Verification items for the finished model (mm, model axes). A direction names the side the tool comes from. Coordinates: 2 decimals unless noted, no trailing zeros. Write each loop counter-clockwise with the first axis right and the second up, starting at its lowest first coordinate (ties: lowest second). Pieces come first, ordered by that corner, then holes. Notation, with made-up numbers: M -15.75,-40 L 26.25,-40 A12 cw 26.25,-18 Z; hole C 71.5,-1 d10. An arc over 180 degrees is marked long. One line per item, written item: value.
```python
from build123d import *

# Parameters (mm, degrees)
CROQUIS1_W                 = 45
CROQUIS1_H                 = 45
SALIENTE_EXTRUIR1_DEPTH    = 300
CROQUIS4_W                 = 18
CROQUIS4_H                 = 34
CORTAR_EXTRUIR2_DEPTH      = 46
CROQUIS8_W                 = 35
CROQUIS8_H                 = 35
CORTAR_EXTRUIR3_DEPTH      = 301
CROQUIS9_W                 = 35
CROQUIS9_H                 = 21.174410022
CORTAR_EXTRUIR4_DEPTH      = 10
CROQUIS10_R                = 1
CORTAR_EXTRUIR5_DEPTH      = 10
CROQUIS11_W                = 45
CROQUIS11_H                = 26.387879272
CORTAR_EXTRUIR6_DEPTH      = 46
CROQUIS13_W                = 45
CROQUIS13_H                = 50
CORTAR_EXTRUIR7_DEPTH      = 23.5
CORTAR_EXTRUIR7_DEPTH_BACK = 23.5
CROQUIS14_W                = 55
CROQUIS14_H                = 55
SALIENTE_EXTRUIR2_DEPTH    = 5
CROQUIS16_R                = 1
CORTAR_EXTRUIR8_DEPTH      = 1
CORTAR_EXTRUIR8_DEPTH_BACK = 229.612120728
CROQUIS17_R                = 2.5
CROQUIS17_R_2              = 2.03
CROQUIS17_R_3              = 1.793308219
CORTAR_EXTRUIR9_DEPTH      = 6
CORTAR_EXTRUIR9_DEPTH_BACK = 51


with BuildPart() as part:
    # Croquis1 → Saliente-Extruir1 (new body)
    with BuildSketch(Plane(origin=(0, 0, 0), x_dir=(1, 0, 0), z_dir=(0, 1, 0))):
        Rectangle(CROQUIS1_W, CROQUIS1_H)
    extrude(amount=SALIENTE_EXTRUIR1_DEPTH)

    # Croquis4 → Cortar-Extruir2 (cut, through all)
    with BuildSketch(Plane.ZY.offset(22.5)):
        with Locations((13.5, 17)):
            Rectangle(CROQUIS4_W, CROQUIS4_H)
    extrude(amount=-CORTAR_EXTRUIR2_DEPTH, mode=Mode.SUBTRACT)

    # Croquis8 → Cortar-Extruir3 (cut, through all)
    with BuildSketch(Plane(origin=(0, 300, 0), x_dir=(1, 0, 0), z_dir=(0, 1, 0))):
        Rectangle(CROQUIS8_W, CROQUIS8_H)
    extrude(amount=-CORTAR_EXTRUIR3_DEPTH, mode=Mode.SUBTRACT)

    # Croquis9 → Cortar-Extruir4 (cut)
    with BuildSketch(Plane(origin=(0, 0, -22.5), x_dir=(-1, 0, 0), z_dir=(0, 0, -1))):
        with Locations((0, 260)):
            Rectangle(CROQUIS9_W, CROQUIS9_H)
    extrude(amount=-CORTAR_EXTRUIR4_DEPTH, mode=Mode.SUBTRACT)

    # Croquis10 → Cortar-Extruir5 (cut)
    with BuildSketch(Plane.XY.offset(22.5)):
        with Locations((0, 260)):
            Circle(CROQUIS10_R)
    extrude(amount=-CORTAR_EXTRUIR5_DEPTH, mode=Mode.SUBTRACT)

    # Croquis11 → Cortar-Extruir6 (cut, through all)
    with BuildSketch(Plane.XY.offset(22.5)):
        with Locations((0, 286.806060364)):
            Rectangle(CROQUIS11_W, CROQUIS11_H)
    extrude(amount=-CORTAR_EXTRUIR6_DEPTH, mode=Mode.SUBTRACT)

    # Croquis13 → Cortar-Extruir7 (cut, two sides)
    with BuildSketch(Plane(origin=(0, 0, 0), x_dir=(0, 0, -1), z_dir=(1, 0, 0))) as cortar_extruir7_sk:
        with Locations((0, 25)):
            Rectangle(CROQUIS13_W, CROQUIS13_H)
    extrude(amount=CORTAR_EXTRUIR7_DEPTH, mode=Mode.SUBTRACT)
    extrude(cortar_extruir7_sk.sketch, amount=-CORTAR_EXTRUIR7_DEPTH_BACK, mode=Mode.SUBTRACT)

    # Croquis14 → Saliente-Extruir2 (add)
    with BuildSketch(Plane.XZ.offset(-50)):
        Rectangle(CROQUIS14_W, CROQUIS14_H)
    extrude(amount=SALIENTE_EXTRUIR2_DEPTH)

    # Croquis16 → Cortar-Extruir8 (cut, two sides)
    with BuildSketch(Plane.XZ.offset(-45)) as cortar_extruir8_sk:
        with Locations((25, 25)):
            Circle(CROQUIS16_R)
        with Locations((-25, 25)):
            Circle(CROQUIS16_R)
        with Locations((-25, -25)):
            Circle(CROQUIS16_R)
        with Locations((25, -25)):
            Circle(CROQUIS16_R)
    extrude(amount=CORTAR_EXTRUIR8_DEPTH, mode=Mode.SUBTRACT)
    extrude(cortar_extruir8_sk.sketch, amount=-CORTAR_EXTRUIR8_DEPTH_BACK, mode=Mode.SUBTRACT)

    # Croquis17 → Cortar-Extruir9 (cut, two sides)
    with BuildSketch(Plane.XY.offset(22.5)) as cortar_extruir9_sk:
        with Locations((-10, 262.50260741)):
            Circle(CROQUIS17_R)
        with Locations((-10, 254.10260741)):
            Circle(CROQUIS17_R_2)
        with Locations((-10, 214.90260741)):
            Circle(CROQUIS17_R_3)
        with Locations((-10, 206.50260741)):
            Circle(CROQUIS17_R)
        with Locations((10, 262.50260741)):
            Circle(CROQUIS17_R)
        with Locations((10, 206.50260741)):
            Circle(CROQUIS17_R)
    extrude(amount=CORTAR_EXTRUIR9_DEPTH, mode=Mode.SUBTRACT)
    extrude(cortar_extruir9_sk.sketch, amount=-CORTAR_EXTRUIR9_DEPTH_BACK, mode=Mode.SUBTRACT)


solid = part.part
```
Item 1: Cross-section at D-D, the plane z = 20.5. Enter the section's corners in (x, y).
The answers:
outline: M -27.5,45 L 27.5,45 L 27.5,50 L 22.5,50 L 22.5,273.61 L -22.5,273.61 L -22.5,50 L -27.5,50 Z; hole C -10,206.5 d5; hole C -10,262.5 d5; hole C -10,254.1 d4.06; hole C -10,214.9 d3.59; hole C 0,260 d2; hole C 10,206.5 d5; hole C 10,262.5 d5
Item 2: Cross-section at B-B, the plane x = 10. Enter the section's corners in (y, z).
The answers:
outline: M 45,-27.5 L 50,-27.5 L 50,-22.5 L 204,-22.5 L 204,-17.5 L 50,-17.5 L 50,17.5 L 204,17.5 L 204,22.5 L 50,22.5 L 50,27.5 L 45,27.5 Z; M 209,-22.5 L 249.41,-22.5 L 249.41,-17.5 L 209,-17.5 Z; M 209,17.5 L 260,17.5 L 260,22.5 L 209,22.5 Z; M 265,17.5 L 273.61,17.5 L 273.61,22.5 L 265,22.5 Z; M 270.59,-22.5 L 273.61,-22.5 L 273.61,-17.5 L 270.59,-17.5 Z
Item 3: Draft check along Y on faces 1 (the face through (11.154, 204.285, 20.035)), 2 (the face through (0, 160, -22.5)), 3 (the face through (20, 273.612, 0)). Enter one of: released by +Y, released by -Y, zero draft, split by the parting line, or undercut.
The answers:
face 1: undercut
face 2: zero draft
face 3: released by +Y
Item 4: Go/stop test with flat-tipped pins: P1, Ø2, axis at y = 147.5, z = -10, coming from the +X side; P2, Ø6, axis at x = 11.5, z = 1, coming from the +Y side; P3, Ø4, axis at x = -10, y = 262.5, coming from the -Z side; P4, Ø12, axis at x = 16, y = 200.5, coming from the -Z side. Record where each tip stops, or that it passes through.
The answers:
P1: stops at x = 22.5
P2: stops at y = 50
P3: passes through
P4: stops at z = -22.5
Item 5: Cross-section at A-A, the plane y = 121. Enter the section's corners in (x, z), and give its area (3 significant figures).
The answers:
outline: M -22.5,-22.5 L 22.5,-22.5 L 22.5,22.5 L -22.5,22.5 Z; hole M -17.5,-17.5 L 17.5,-17.5 L 17.5,17.5 L -17.5,17.5 Z
area: 800 mm²
Item 6: Cross-section at C-C, the plane z = 11. Enter the section's corners in (x, y), and give its area (3 significant figures).
The answers:
outline: M -27.5,45 L 27.5,45 L 27.5,50 L 22.5,50 L 22.5,273.61 L 17.5,273.61 L 17.5,50 L -17.5,50 L -17.5,273.61 L -22.5,273.61 L -22.5,50 L -27.5,50 Z
area: 2,510 mm²
Item 7: Scan lines: line 1 (Y direction, x = -10, z = -20.5); line 2 (Z direction, x = -25, y = 46); line 3 (Y direction, x = 10, z = 21.35). Record each from-to range of solid material in increasing order.
The answers:
line 1: y = 45 to 204, 209 to 213.11, 216.7 to 249.41, 270.59 to 273.61
line 2: z = -27.5 to -26, -24 to 24, 26 to 27.5
line 3: y = 45 to 204, 209 to 260, 265 to 273.61
Item 8: Access from +Z, -Z, +X, -X, +Y, -Y to the whole of each face (thin tool, end or side, straight path). Record for faces 4 (the face through (-22.5, 160, 0)), 5 (the face through (0, 160, 22.5)), 6 (the face through (22.5, 160, 0)), 7 (the face through (0, 249.413, -20)), 8 (the face through (0, 50, 0)).
The answers:
face 4: +Z, -Z, -X, +Y
face 5: +Z, +X, -X, +Y
face 6: +Z, -Z, +X, +Y
face 7: -Z
face 8: +Y
